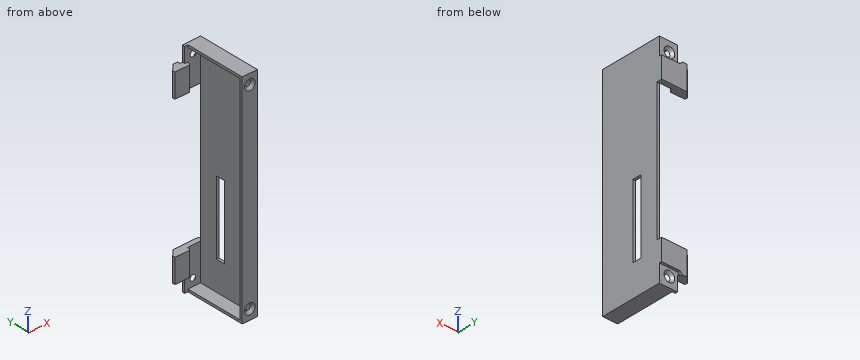
Autodesk Inventor part; units mm, degrees
ref_plane "YZ Plane" through (0, 0, 0) normal (1, 0, 0) x (0, 1, 0)
ref_plane "XZ Plane" through (0, 0, 0) normal (0, 1, 0) x (-1, 0, 0)
ref_plane "XY Plane" through (0, 0, 0) normal (0, 0, 1) x (1, 0, 0)
sketch "Sketch1" plane through (0, 0, 0) normal (1, 0, 0) x (0, 1, 0)
  line L0 (0, 0) -> (-47.4, 0)
  line L1 (-47.4, 0) -> (-47.4, 172)
  line L2 (-47.4, 172) -> (0, 172)
  line L3 (0, 172) -> (0, 0)
  dimension "d0" = 172
  dimension "d1" = 47.4
extrude "Extrusion1" add sketch "Sketch1" along normal blind 2
sketch "Sketch2" plane through (0, 0, 0) normal (-1, 0, 0) x (0, 0, 1)
  line L0 (0, 0) -> (172, 0)
  line L1 (172, -47.4) -> (0, -47.4)
  line L2 (0, 0) -> (2, 0)
  line L3 (2, 0) -> (2, -47.4)
  line L4 (2, -47.4) -> (0, -47.4)
  line L5 (0, -47.4) -> (0, 0)
  line L6 (172, 0) -> (172, -47.4)
  line L7 (0, -47.4) -> (172, -47.4)
  line L8 (172, -47.4) -> (172, -45.4)
  line L9 (172, -45.4) -> (0, -45.4)
  line L10 (0, -45.4) -> (0, -47.4)
  line L11 (172, -47.4) -> (170, -47.4)
  line L12 (170, -47.4) -> (170, 0)
  line L13 (170, 0) -> (172, 0)
  line L14 (172, 0) -> (172, -47.4)
  point P0 (2, -45.4)
  point P1 (0, -47.4)
  point P2 (170, -45.4)
  dimension "d4" = 2
  dimension "d5" = 2
  dimension "d6" = 2
extrude "Extrusion2" add sketch "Sketch2" along normal blind 10 contours L0 L3 L9 L5 | L9 L3 L1 L5 | L0 L6 L9 L12 | L9 L12 L1 L3 | L9 L6 L1 L12
sketch "Sketch3" plane through (2, 0, 172) normal (0, 1, 0) x (1, 0, 0)
  line L0 (0, 0) -> (0, 172)
  line L1 (0, 12) -> (-25, 12)
  line L2 (-25, 12) -> (-25, 31)
  line L3 (-25, 31) -> (0, 31)
  line L4 (0, 31) -> (0, 12)
  line L5 (-12, 0) -> (0, 0)
  point P0 (-2, 172)
  point P1 (0, 31)
  dimension "d9" = 12
  dimension "d10" = 25
  dimension "d11" = 19
extrude "Extrusion3" add sketch "Sketch3" along normal blind 4
sketch "Sketch4" plane through (2, 0, 172) normal (0, -1, 0) x (1, 0, 0)
  line L0 (-2, -31) -> (-2, -12)
  line L1 (0, -12) -> (0, -31)
  line L2 (0, -31) -> (-25, -31)
  line L3 (-25, -31) -> (-25, -12)
  line L4 (-25, -12) -> (0, -12)
  line L5 (-25, -31) -> (-25, -12)
  line L6 (-2, -31) -> (-25, -31)
  line L7 (-25, -12) -> (-12.388, -12)
  line L8 (-12.388, -12) -> (-12.388, -31)
  line L9 (-12.388, -31) -> (-25, -31)
  line L10 (-25, -31) -> (-25, -12)
  point P0 (-2, -172)
  point P1 (-12.388, -12)
  dimension "d14" = 12.388
extrude "Extrusion4" add sketch "Sketch4" along normal blind 3 contours L2 L3 L4 L8
chamfer "Chamfer1" distance 1 angle 45 1 edges at (-10.388, -3, 150.5)
chamfer "Chamfer2" distance 5 angle 45 1 edges at (-23, 4, 150.5)
sketch "Sketch5" plane through (0, 0, 160) normal (0, 0, 1) x (1, 0, 0)
  line L0 (0, 0) -> (-10, 0)
  line L1 (2, 0) -> (-12.5, 0)
  line L2 (-12.5, 0) -> (-12.5, 2)
  line L3 (-12.5, 2) -> (2, 2)
  line L4 (2, 2) -> (2, 0)
  point P0 (-5, 0)
  dimension "d26" = 14.5
  dimension "d27" = 2
extrude "Extrusion5" add sketch "Sketch5" along normal up to surface (12 mm away)
ref_plane "Work Plane1" through (-10, -47.4, 86) normal (0, 0, 1) x (1, 0, 0)
sketch "Sketch6" plane through (-12.5, 2, 160) normal (0, 1, 0) x (1, 0, 0)
  line L0 (0, -12) -> (14.5, -12)
  line L1 (14.5, 0) -> (14.5, -12)
  point P0 (12.5, 160)
  point P1 (6.5, -4)
  dimension "d28" = 8
  dimension "d29" = 8
hole "Hole1" at (-6, 2, 164) direction (0, -1, 0) diameter 4 depth 10 tip angle 118 countersink diameter 8.4 countersink angle 90
sketch "Sketch7" plane through (2, 4, 172) normal (0, 1, 0) x (1, 0, 0)
  line L0 (-20, 12) -> (0, 12)
  line L1 (0, 12) -> (-14.5, 12)
  line L2 (-14.5, 12) -> (-14.5, 14)
  line L3 (-14.5, 14) -> (0, 14)
  line L4 (0, 14) -> (0, 12)
  point P0 (-2, 172)
  dimension "d37" = 14.5
  dimension "d38" = 2
extrude "Extrusion6" cut sketch "Sketch7" against normal up to surface (2 mm away)
chamfer "Chamfer3" distance 2 angle 45 1 edges at (-12.5, 3, 160)
mirror "Mirror2" about plane through (-10, -47.4, 86) normal (0, 0, 1) of "Extrusion3", "Extrusion5", "Hole1", "Chamfer3", "Chamfer2", "Chamfer1", "Extrusion4", "Extrusion6"
sketch "Sketch8" plane through (2, -47.4, 0) normal (0, -1, 0) x (1, 0, 0)
  circle A0 centre (-8, 164) radius 2.2
  circle A1 centre (-8, 164) radius 4.2
  circle A2 centre (-8, 8) radius 4.2
  circle A3 centre (-8, 8) radius 2.2
  circle A4 centre (-8, 8) radius 4.2
  line L0 (0, 172) -> (0, 0)
  point P0 (-2, 0)
  point P1 (-12, 2)
  point P2 (-6, 8)
  dimension "d51" = 6
hole "Hole2" at (-4, -47.4, 8) direction (0, 1, 0) diameter 4 depth 10 tip angle 118 countersink diameter 8.4 countersink angle 90
mirror "Mirror3" about plane through (-10, -47.4, 86) normal (0, 0, 1) of "Hole2"
sketch "Sketch9" plane through (2, 0, 0) normal (1, 0, 0) x (0, 0, -1)
  line L0 (0, 2) -> (-14, 2)
  line L1 (0, -47.4) -> (0, 2)
  line L2 (-31, 0) -> (-141, 0)
  line L3 (-25, -14) -> (-83, -14)
  line L4 (-83, -14) -> (-83, -21)
  line L5 (-83, -21) -> (-25, -21)
  line L6 (-25, -21) -> (-25, -14)
  point P0 (0, 0)
  point P1 (-83, -14)
  dimension "d52" = 16
  dimension "d53" = 25
  dimension "d54" = 14
  dimension "d55" = 58
  dimension "d56" = 7
extrude "Extrusion7" cut sketch "Sketch9" against normal blind 10
properties part number "backplate"
For this review, take the finished solid that the model builds, in its own axes (mm). Coordinates: 2 decimals unless noted, no trailing zeros. Order: outer loops, then holes, each group sorted by start corner. A loop starts at its lowest first (then second) coordinate and runs counter-clockwise, first axis right, second up. Notation, with made-up numbers: (40, 50) -> (86, 50) arc R18 cw to (86, 78) -> close; hole circle Ø4 at (-39.75, 82.5). An arc over 180 degrees is marked (long way). Answer as CSV lines item,"result".
Q1. We need section A-A (y = -16). State the section outline as (x, z) points.
Model answer:
outline,"(-10, 0) -> (2, 0) -> (2, 25) -> (0, 25) -> (0, 2) -> (-10, 2) -> close; (-10, 170) -> (0, 170) -> (0, 83) -> (2, 83) -> (2, 172) -> (-10, 172) -> close"
Q2. We need section C-C (z = 8). State the section outline as (x, y) points.
Model answer:
outline,"(-12.5, 0) -> (-8.2, 0) -> (-10.2, 2) -> (-12.5, 2) -> close; (-10, -47.4) -> (-8.2, -47.4) -> (-6.2, -45.4) -> (-10, -45.4) -> close; (-3.8, 0) -> (0, 0) -> (0, -45.4) -> (-1.8, -45.4) -> (0.2, -47.4) -> (2, -47.4) -> (2, 2) -> (-1.8, 2) -> close"
Q3. We need section B-B (x = -16.25). State the section outline as (y, z) points, plus the area to 3 significant figures.
Model answer:
outline,"(-3, 12) -> (4, 12) -> (4, 31) -> (-3, 31) -> close; (-3, 141) -> (4, 141) -> (4, 160) -> (-3, 160) -> close"
area,"266 mm2"
Q4. We need section D-D (y = -41.5). State the section outline as (x, z) points.
Model answer:
outline,"(-10, 0) -> (2, 0) -> (2, 172) -> (-10, 172) -> (-10, 170) -> (0, 170) -> (0, 2) -> (-10, 2) -> close"
Q5. Clearance check with flat-ended pins moving along their axes: pin 1 Ø1 at (x, z) = (0.5, 52.5) entering from +Y; pin 2 Ø8 at (y, z) = (-12.5, 141) entering from -X; pin 3 Ø1 at (y, z) = (1, 166) entering from -X; pin 4 Ø12 at (x, y) = (-17.5, -17.5) entering from +Z. State where each tip first meets the part, or that it passes through.
Model answer:
pin 1,"stops at y = 0"
pin 2,"stops at x = 0"
pin 3,"stops at x = -12.5"
pin 4,"passes through"
Q6. Wall thickness on line 1 along Z through (x, y) = (-1.5, 1); line 2 along Z through (x, y) = (-8, -23.5); line 3 along Y through (x, z) = (-4.75, 27): over which ranges is each line inside the solid? List them lowest first. Write a range as [from, to].
Model answer:
line 1,"z = [0, 31], [141, 172]"
line 2,"z = [0, 2], [170, 172]"
line 3,"y = [-47.4, -45.4], [0, 4]"
